Read the model definition and answer for the solid it produces. Units are mm, in the model's axes. Round coordinates to 2 decimals unless told otherwise and drop trailing zeros. Order: outer loops, then holes, each group sorted by start corner. A loop starts at its lowest first (then second) coordinate and runs counter-clockwise, first axis right, second up.
Autodesk Inventor part; units mm, degrees
ref_plane "YZ Plane" through (0, 0, 0) normal (1, 0, 0) x (0, 1, 0)
ref_plane "XZ Plane" through (0, 0, 0) normal (0, 1, 0) x (-1, 0, 0)
ref_plane "XY Plane" through (0, 0, 0) normal (0, 0, 1) x (1, 0, 0)
sketch "Esboço1" plane through (0, 0, 0) normal (0, 0, 1) x (1, 0, 0)
  line L0 (0, 0) -> (70, 0)
  line L1 (70, 0) -> (70, 35)
  line L2 (70, 35) -> (0, 35)
  line L3 (0, 35) -> (0, 0)
  dimension "d0" = 70
  dimension "d1" = 35
extrude "Extrusão1" add sketch "Esboço1" along normal blind 10
fillet "Arredondamento1" radius 3 4 edges at (70, 35, 5) (70, 0, 5) (0, 35, 5) (0, 0, 5)
fillet "Arredondamento2" radius 3 8 edges at (0.8787, 34.1213, 0) (0, 17.5, 0) (0.8787, 0.8787, 0) (35, 0, 0) (69.1213, 0.8787, 0) (70, 17.5, 0) (69.1213, 34.1213, 0) (35, 35, 0)
sketch "Esboço3" plane through (0, 0, 0) normal (0, 0, -1) x (-1, 0, 0)
  line L0 (-3, 35) -> (-67, 35)
  line L1 (-67, 3) -> (-67, 32)
  line L2 (-67, 0) -> (-3, 0)
  line L3 (-3, 32) -> (-3, 3)
  point P0 (0, 0)
  point P1 (-57, 25)
  point P2 (-13, 25)
  point P3 (-13, 10)
  point P4 (-57, 10)
  dimension "d18" = 10
  dimension "d19" = 10
  dimension "d20" = 10
  dimension "d21" = 10
  dimension "d22" = 10
  dimension "d23" = 10
  dimension "d24" = 10
  dimension "d25" = 10
hole "Furo1" at (57, 25, 0) at (13, 25, 0) at (13, 10, 0) at (57, 10, 0) direction (0, 0, 1) diameter 3 end through all
thread "Rosca1"
thread "Rosca2"
thread "Rosca3"
thread "Rosca4"
properties part number "Peça4-Rubia"
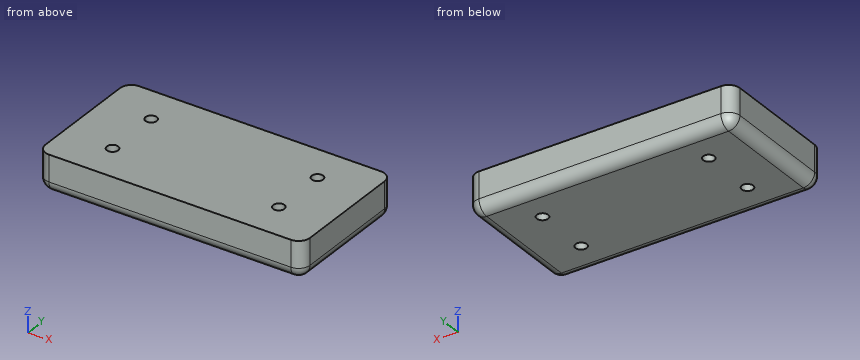
Q1. A flat-ended cylindrical pin translates along its axis: pin 1 (1.8 mm diameter, centred on x = 57, y = 10, fed in from -Z). Find the tip coordinate at first contact, or state that the pin passes through.
Outcome:
pin 1: passes through
Q2. A cutting plane is placed at A-A, the plane x = 57. Give the vertices of the cut face in (y, z), plus the area to 3 significant figures.
Outcome:
outline: (0, 3) arc R3 ccw to (3, 0) - (8.5, 0) - (8.5, 10) - (0, 10) - close; (11.5, 0) - (23.5, 0) - (23.5, 10) - (11.5, 10) - close; (26.5, 0) - (32, 0) arc R3 ccw to (35, 3) - (35, 10) - (26.5, 10) - close
area: 286 mm2
Q3. A cutting plane is placed at B-B, the plane y = 10. Give the vertices of the cut face in (x, z), plus the area to 3 significant figures.
Outcome:
outline: (0, 3) arc R3 ccw to (3, 0) - (11.5, 0) - (11.5, 10) - (0, 10) - close; (14.5, 0) - (55.5, 0) - (55.5, 10) - (14.5, 10) - close; (58.5, 0) - (67, 0) arc R3 ccw to (70, 3) - (70, 10) - (58.5, 10) - close
area: 636 mm2
Q4. A cutting plane is placed at C-C, the plane y = 33.5. Give the vertices of the cut face in (x, z), plus the area to 3 significant figures.
Outcome:
outline: (0.4, 3) arc R2.6 ccw to (3, 0.4) - (67, 0.4) arc R2.6 ccw to (69.6, 3) - (69.6, 10) - (0.4, 10) - close
area: 661 mm2
Q5. Straight lines are drawn through the part: probe 1 along X at (y, z) = (25, 4.75); probe 2 along Y at (x, z) = (57, 3.5); probe 3 along X at (y, z) = (26, 2). For each, find the intervals that lie inside material, in ascending order.
Outcome:
probe 1: x = 0 to 11.5, 14.5 to 55.5, 58.5 to 70
probe 2: y = 0 to 8.5, 11.5 to 23.5, 26.5 to 35
probe 3: x = 0.17 to 11.88, 14.12 to 55.88, 58.12 to 69.83
